Verification items for the finished model (mm, model axes). Face numbers are marked on the shaded views. Coordinates: 2 decimals unless noted, no trailing zeros. Write each loop counter-clockwise with the first axis right and the second up, starting at its lowest first coordinate (ties: lowest second). Pieces come first, ordered by that corner, then holes. Notation, with made-up numbers: (45.5, 62) -> (97.5, 62) arc R29 ccw to (97.5, 82) -> close; hole circle Ø9 at (-31.5, 18.25). An arc over 180 degrees is marked (long way). Use CSV: the item, a comma, the result in double quotes.
```python
from build123d import *

# Parameters (mm, degrees)
SKETCH1_R               = 25
BOSS_EXTRUDE1_DEPTH     = 50
SKETCH2_R               = 3
CUT_EXTRUDE1_DEPTH      = 20
SKETCH3_R               = 4
CUT_EXTRUDE2_DEPTH      = 30
CUT_EXTRUDE3_DEPTH      = 62.23724357
CUT_EXTRUDE3_DEPTH_BACK = 62.23724357
SKETCH4_R               = 2


with BuildPart() as part:
    # Sketch1 → Boss-Extrude1 (new body)
    with BuildSketch(Plane.XY):
        Circle(SKETCH1_R)
    extrude(amount=BOSS_EXTRUDE1_DEPTH)

    # Sketch2 → Cut-Extrude1 (cut)
    with BuildSketch(Plane.XY.offset(50)):
        Circle(SKETCH2_R)
    extrude(amount=-CUT_EXTRUDE1_DEPTH, mode=Mode.SUBTRACT)

    # Sketch3 → Cut-Extrude2 (cut)
    with BuildSketch(Plane(origin=(0, 0, 0), x_dir=(-1, 0, 0), z_dir=(0, 0, -1))):
        Circle(SKETCH3_R)
    extrude(amount=-CUT_EXTRUDE2_DEPTH, mode=Mode.SUBTRACT)

    # Sketch4 → Cut-Extrude3 (cut, two sides: drawn at the far end of the back side and taken through both)
    with BuildSketch(Plane(origin=(0, 0, 0), x_dir=(0, 0, -1), z_dir=(1, 0, 0)).offset(-CUT_EXTRUDE3_DEPTH_BACK)):
        with Locations((-43.847378844, 0)):
            Circle(SKETCH4_R)
        with Locations((-6.152621156, 0)):
            Circle(SKETCH4_R)
    extrude(amount=CUT_EXTRUDE3_DEPTH + CUT_EXTRUDE3_DEPTH_BACK, mode=Mode.SUBTRACT)


solid = part.part
```
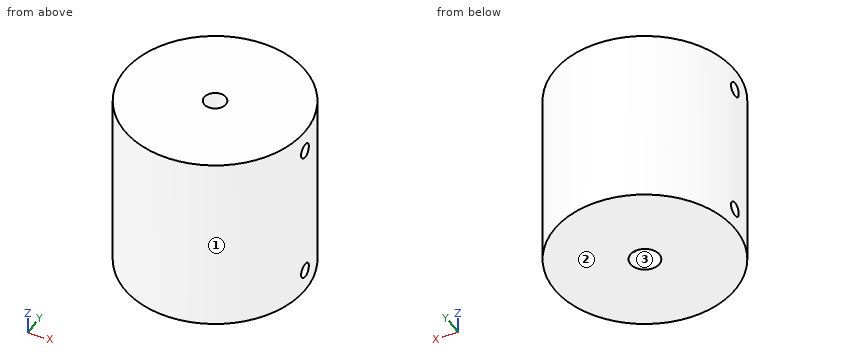
1) Mould release check, pull along X, two halves, no side actions. Record for the marked faces 1, 2 and 3: released by +X, released by -X, zero draft, split by the parting line, or undercut.
Return value:
face 1,"split by the parting line"
face 2,"zero draft"
face 3,"undercut"
2) Scan lines: L1, parallel to X at y = 0, z = 38.75; L2, parallel to X at y = -3, z = 13.5; L3, parallel to Y at x = -5, z = 13. Record each from-to range of solid material in increasing order.
Return value:
L1,"-25 to -3, 3 to 25"
L2,"-24.82 to -2.65, 2.65 to 24.82"
L3,"-24.49 to 24.49"
3) Cross-section at A-A (y = 0). Record the boundary of the cut face in (x, z).
Return value:
outline,"(-25, 0) -> (-4, 0) -> (-4, 4.15) -> (-25, 4.15) -> close; (-25, 8.15) -> (-4, 8.15) -> (-4, 30) -> (-3, 30) -> (-3, 41.85) -> (-25, 41.85) -> close; (-25, 45.85) -> (-3, 45.85) -> (-3, 50) -> (-25, 50) -> close; (3, 30) -> (4, 30) -> (4, 8.15) -> (25, 8.15) -> (25, 41.85) -> (3, 41.85) -> close; (3, 45.85) -> (25, 45.85) -> (25, 50) -> (3, 50) -> close; (4, 0) -> (25, 0) -> (25, 4.15) -> (4, 4.15) -> close"
4) Cross-section at B-B (x = 0). Record the boundary of the cut face in (y, z).
Return value:
outline,"(-25, 0) -> (-4, 0) -> (-4, 30) -> (-3, 30) -> (-3, 50) -> (-25, 50) -> close; (3, 30) -> (4, 30) -> (4, 0) -> (25, 0) -> (25, 50) -> (3, 50) -> close"
5) Gauge pin test, flat ends, axial feed: pin 1 (12 mm diameter, centred on x = 16, y = 18, fed in from -Z); pin 2 (8 mm diameter, centred on x = 2, z = 36, fed in from +Y); pin 3 (10 mm diameter, centred on x = -10.5, z = 15, fed in from +Y); pin 4 (2.5 mm diameter, centred on x = 0.5, y = 1.5, fed in from -Z). Record the tip position at first contact, or that the pin passes through.
Return value:
pin 1,"z = 0"
pin 2,"y = 25"
pin 3,"y = 24.39"
pin 4,"through"
6) Cross-section at D-D (x = -9). Record the boundary of the cut face in (y, z).
Return value:
outline,"(-23.32, 0) -> (23.32, 0) -> (23.32, 50) -> (-23.32, 50) -> close; hole circle Ø4 at (0, 6.15); hole circle Ø4 at (0, 43.85)"
7) Cross-section at C-C (z = 18.5). Record the boundary of the cut face in (x, y), plus the area to 3 significant figures.
Return value:
outline,"circle Ø50 at (0, 0); hole circle Ø8 at (0, 0)"
area,"1,910 mm2"
